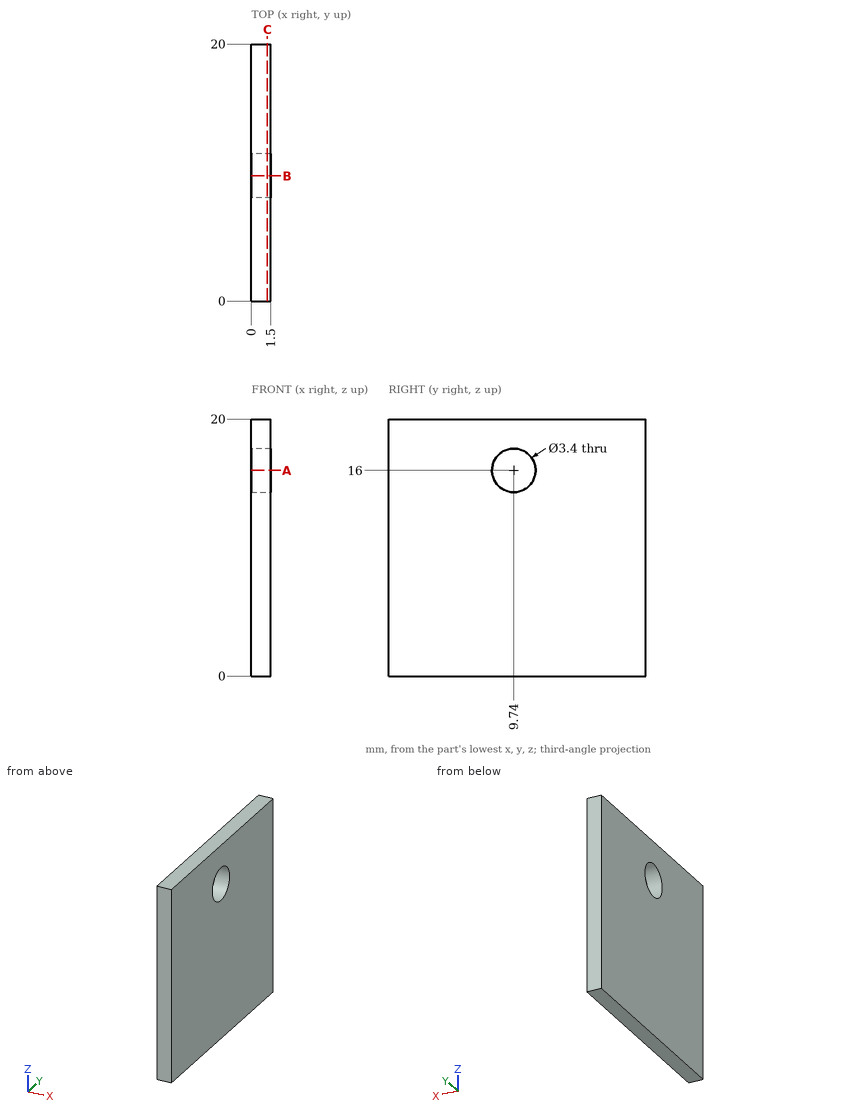
Could you check a few things on this drawing? It's one solid part, dimensions in mm from its lowest x, y, z. Coordinates: 2 decimals unless noted, no trailing zeros. Loops run counter-clockwise (first coordinate to the right, second up) from the corner with the lowest first, then second, coordinate; pieces in that order, holes last.
1. For P1, Ø3, axis at y = 9.74, z = 16, coming from the -X side, with a flat end and sliding along its axis, tell me the tip position at first contact or that it passes through.
2. I need wall thicknesses on L1, parallel to Z at x = 0.85, y = 9.74; L2, parallel to Y at x = 0.4, z = 16; L3, parallel to Z at x = 0.3, y = 11.25. Which ranges of each line are inside material? Lowest first, please.
3. Imagine slicing it at C-C (x = 1.25). Please give me the cut outline in (y, z).
4. Imagine slicing it at A-A (z = 16). Please give me the cut outline in (x, y), and give its area (3 significant figures).
5. Imagine slicing it at B-B (y = 9.74). Please give me the cut outline in (x, z), and give its area (3 significant figures).
Computed values:
1. P1: passes through
2. L1: z = 0 to 14.3, 17.7 to 20
2. L2: y = 0 to 8.04, 11.44 to 20
2. L3: z = 0 to 15.22, 16.78 to 20
3. outline: (0, 0) - (20, 0) - (20, 20) - (0, 20) - close; hole circle Ø3.4 at (9.74, 16)
4. outline: (0, 0) - (1.5, 0) - (1.5, 8.04) - (0, 8.04) - close; (0, 11.44) - (1.5, 11.44) - (1.5, 20) - (0, 20) - close
4. area: 24.9 mm2
5. outline: (0, 0) - (1.5, 0) - (1.5, 14.3) - (0, 14.3) - close; (0, 17.7) - (1.5, 17.7) - (1.5, 20) - (0, 20) - close
5. area: 24.9 mm2
